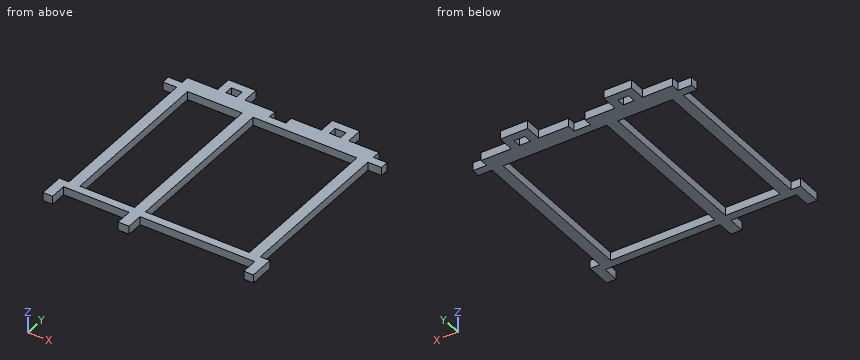
from build123d import *

# Parameters (mm, degrees)
SKETCH1_W           = 20
SKETCH1_H           = 59
SKETCH1_W_2         = 38
BOSS_EXTRUDE1_DEPTH = 3
BOSS_EXTRUDE2_DEPTH = 3


with BuildPart() as part:
    # Sketch1 → Boss-Extrude1 (new body)
    with BuildSketch(Plane.XY):
        Polygon((5, -3), (0, -3), (0, 0), (5, 0), (5, 3), (37, 3), (37, 0), (43, 0), (43, 3), (75, 3), (75, 0), (80, 0), (80, -3), (75, -3), (75, -62), (78.5, -62), (78.5, -71), (75, -71), (75, -65), (33, -65), (33, -71), (29, -71), (29, -65), (5, -65), (5, -71), (1.5, -71), (1.5, -62), (5, -62), align=None)
        with Locations((19, -32.5)):
            Rectangle(SKETCH1_W, SKETCH1_H, mode=Mode.SUBTRACT)
        with Locations((52, -32.5)):
            Rectangle(SKETCH1_W_2, SKETCH1_H, mode=Mode.SUBTRACT)
    extrude(amount=BOSS_EXTRUDE1_DEPTH)

    # Sketch2 → Boss-Extrude2 (add)
    with BuildSketch(Plane.XY.offset(3)):
        Polygon((16, 9), (16, 3), (19, 3), (19, 6), (23, 6), (23, 3), (26, 3), (26, 9), align=None)
        Polygon((54, 3), (57, 3), (57, 6), (61, 6), (61, 3), (64, 3), (64, 9), (54, 9), align=None)
    extrude(amount=-BOSS_EXTRUDE2_DEPTH)


solid = part.part
Could you check a few things on this model? Use its own coordinates, in mm. Coordinates: 2 decimals unless noted, no trailing zeros. Order: outer loops, then holes, each group sorted by start corner. A loop starts at its lowest first (then second) coordinate and runs counter-clockwise, first axis right, second up. Notation, with made-up numbers: (-30, -30.5) -> (-13, -30.5) arc R22 ccw to (-13, -18.5) -> close; hole circle Ø3 at (-38.5, 74.5). An arc over 180 degrees is marked (long way). One line per item, written item: value. Start each with the question number.
1) Imagine slicing it at D-D on y = -64. List the corners of the cut face in (x, z) for me, plus the area to 3 significant figures.
2) I'm going to push flat-ended pins straight in: pin 1 (0.9 mm diameter, centred on y = -67, z = 1, fed in from +X); pin 2 (1.5 mm diameter, centred on y = 5, z = 1, fed in from -X); pin 3 (1.5 mm diameter, centred on y = -34, z = 1, fed in from +X); pin 4 (12 mm diameter, centred on x = 46, y = -14.5, fed in from -Z). Where does each tip first touch, or does it pass through?
3) If I drill on L1, parallel to X at y = -35, z = 0.8; L2, parallel to Y at x = 21.5, z = 1.4; L3, parallel to Y at x = 53, z = 2.6, over which ranges is the centre line in solid material (lowest first)? Write a range as [from, to].
4) Imagine slicing it at C-C on x = 50. List the corners of the cut face in (y, z) for me.
5) Imagine slicing it at A-A on x = 17.5. List the corners of the cut face in (y, z) for me, plus the area to 3 significant figures.
6) Imagine slicing it at B-B on y = -55.5. List the corners of the cut face in (x, z) for me.
Answer list:
1. outline: (1.5, 0) -> (78.5, 0) -> (78.5, 3) -> (1.5, 3) -> close
1. area: 231 mm2
2. pin 1: stops at x = 78.5
2. pin 2: stops at x = 16
2. pin 3: stops at x = 75
2. pin 4: passes through
3. L1: x = [5, 9], [29, 33], [71, 75]
3. L2: y = [-65, -62], [-3, 3], [6, 9]
3. L3: y = [-65, -62], [-3, 3]
4. outline: (-65, 0) -> (-62, 0) -> (-62, 3) -> (-65, 3) -> close; (-3, 0) -> (3, 0) -> (3, 3) -> (-3, 3) -> close
5. outline: (-65, 0) -> (-62, 0) -> (-62, 3) -> (-65, 3) -> close; (-3, 0) -> (9, 0) -> (9, 3) -> (-3, 3) -> close
5. area: 45.0 mm2
6. outline: (5, 0) -> (9, 0) -> (9, 3) -> (5, 3) -> close; (29, 0) -> (33, 0) -> (33, 3) -> (29, 3) -> close; (71, 0) -> (75, 0) -> (75, 3) -> (71, 3) -> close
